Study the drawing (mm; zero at the part's minimum x, y, z) and answer. A direction names the side the tool comes from. Coordinates: 2 decimals unless noted, no trailing zeros. Loops run counter-clockwise (first coordinate to the right, second up) from the corner with the lowest first, then second, coordinate; pieces in that order, holes last. Notation, with made-up numbers: (-8, 11.25) -> (3, 11.25) arc R16 ccw to (3, 21.25) -> close; hole circle Ø4 at (47, 53). An arc over 180 degrees is marked (long way). Answer as CSV lines item,"result".
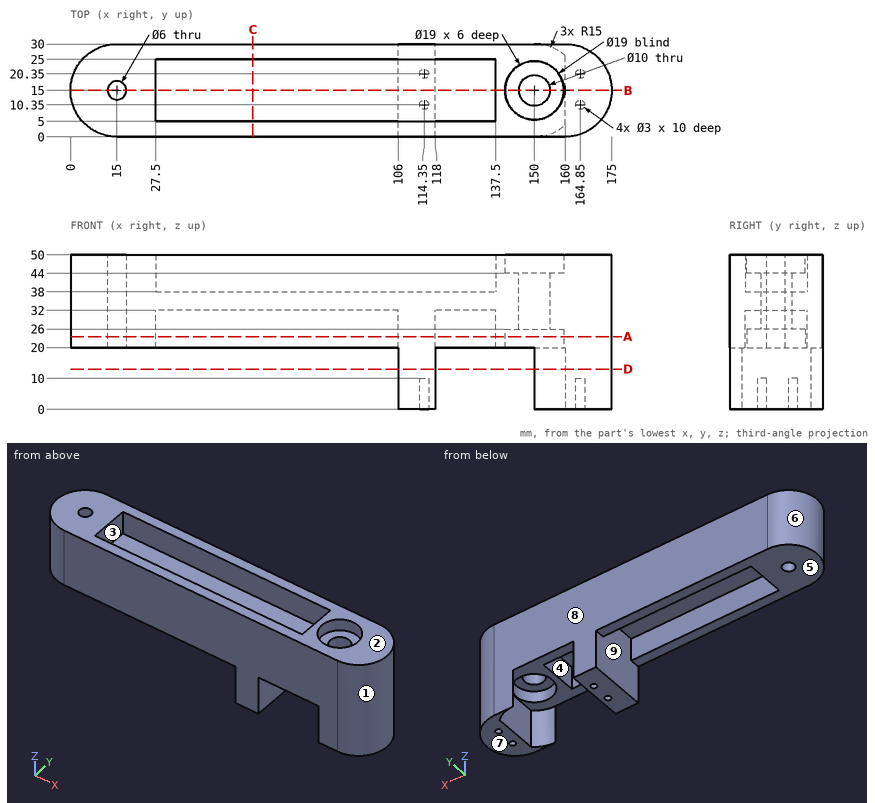
Q1. A cutting plane is placed at A-A, the plane z = 23.5. Write down the section's boundary in (x, y), and give its area (4 significant figures).
Results:
outline,"(15, 0) -> (160, 0) arc R15 ccw to (160, 30) -> (15, 30) arc R15 ccw to start; hole circle Ø6 at (15, 15); hole (27.5, 5) -> (106, 5) -> (106, 25) -> (27.5, 25) -> close; hole (118, 5) -> (137.5, 5) -> (137.5, 25) -> (118, 25) -> close; hole circle Ø19 at (150, 15)"
area,"2,785 mm²"
Q2. Given pin 1 Ø1 at (y, z) = (13, 23.5) entering from -X (3 decimals); pin 2 Ø6 at (y, z) = (12.5, 11.5) entering from -X; pin 3 Ø0.9 at (x, y) = (114, 20) entering from -Z, each flat-ended and moving along its own axis, determine where each tip first touches the part or whether it passes through.
Results:
pin 1,"stops at x = 0.075"
pin 2,"stops at x = 106"
pin 3,"stops at z = 10"
Q3. A cutting plane is placed at C-C, the plane x = 59. Write down the section's boundary in (y, z).
Results:
outline,"(0, 20) -> (5, 20) -> (5, 32) -> (25, 32) -> (25, 20) -> (30, 20) -> (30, 50) -> (25, 50) -> (25, 38) -> (5, 38) -> (5, 50) -> (0, 50) -> close"
Q4. A cutting plane is placed at D-D, the plane z = 13. Write down the section's boundary in (x, y).
Results:
outline,"(106, 0) -> (118, 0) -> (118, 30) -> (106, 30) -> close; (150, 0) -> (160, 0) arc R15 ccw to (160, 30) -> (150, 30) arc R15 cw to (160, 26.18) -> (160, 3.82) arc R15 cw to start"
Q5. For a pull along Y with two mould halves and no side action, classify the marked faces 6, 7, 8 and 9 as pulls with the +Y half, pulls with the -Y half, needs draft (parallel to the pull), parting line crosses it, or undercut.
Results:
face 6,"parting line crosses it"
face 7,"needs draft"
face 8,"pulls with the +Y half"
face 9,"undercut"
Q6. A cutting plane is placed at B-B, the plane y = 15. Give the number of separate pieces and of enclosed holes in the cut face, and give its area (3 significant figures).
Results:
separate pieces,"3"
enclosed holes,"0"
area,"2,710 mm²"
Q7. For the marked faces 1, 2, 3, 4 and 5, determine the directions among +Z, -Z, +X, -X, +Y, -Y from which every point of the face is accessible in a straight line to the end or side of a thin tool.
Results:
face 1,"+Z, -Z, +X"
face 2,"+Z, +X, -X, +Y, -Y"
face 3,"+Z"
face 4,"-Z"
face 5,"-Z, -X, +Y, -Y"
Q8. Find the intervals of material crossed by probe 1 along Y at (x, z) = (114.35, 4.5); probe 2 along X at (y, z) = (15.25, 27); probe 3 along Y at (x, z) = (150, 24), in increasing order. Write a range as [from, to].
Results:
probe 1,"y = [0, 8.85], [11.85, 18.85], [21.85, 30]"
probe 2,"x = [0, 12.01], [17.99, 27.5], [106, 118], [137.5, 145.01], [154.99, 175]"
probe 3,"y = [0, 5.5], [24.5, 30]"
